Can you work these out from the model? Positions are in its coordinate system, mm. Face numbers are marked on the shaded views. A direction names the side the tool comes from. Give positions to 0.01 mm unless a question says otherwise; leave off trailing zeros. Write each loop counter-clockwise with the first axis right and the second up, starting at its lowest first coordinate (ties: lowest second). Pieces come first, ordered by that corner, then holes.
1. Suppose I cut it at A-A (x = 0.75). Please give me the cut outline in (y, z).
2. Suppose I cut it at B-B (y = 2). Please give me the cut outline in (x, z).
3. Suppose I cut it at D-D (z = -16). Please give me the cut outline in (x, y), and give its area (3 significant figures).
4. I'm going to push flat-ended pins straight in: pin 1 (5 mm diameter, centred on y = 12.5, z = -27, fed in from +X); pin 2 (1.5 mm diameter, centred on x = 1.5, z = -4, fed in from +Y). Where does each tip first touch, or does it pass through?
5. On a 3-axis mill with a long thin cutter (end or side, diameter ignored), from which of +Z, -Z, +X, -X, +Y, -Y can I reach the whole of each face in a straight line? I mean the marked faces 1 and 2. Say none if no direction works.
6. Suppose I cut it at C-C (z = -8). Please give me the cut outline in (x, y), and give its area (3 significant figures).
7. If I drill on probe 1 along Z at (x, y) = (1.25, 1.5); probe 2 along X at (y, z) = (11.75, -13), over which ranges is the centre line in solid material (lowest first)?
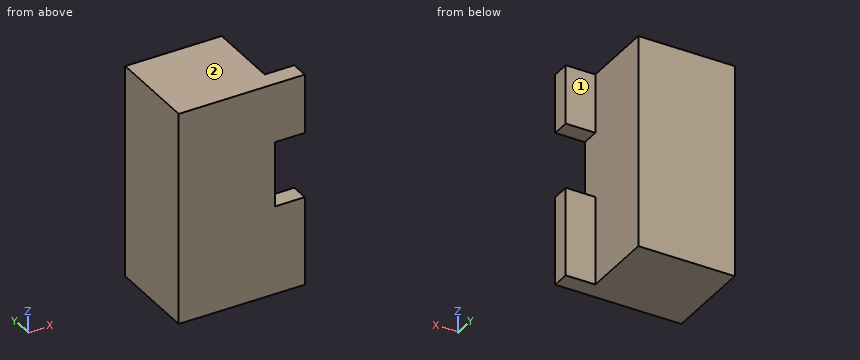
Autodesk Inventor part; units mm, degrees
ref_plane "YZ Plane" through (0, 0, 0) normal (1, 0, 0) x (0, 1, 0)
ref_plane "XZ Plane" through (0, 0, 0) normal (0, 1, 0) x (-1, 0, 0)
ref_plane "XY Plane" through (0, 0, 0) normal (0, 0, 1) x (1, 0, 0)
sketch "Sketch1" plane through (0, 0, 0) normal (0, 1, 0) x (-1, 0, 0)
  line L0 (16.3, 0) -> (0, 0)
  line L1 (0, 0) -> (0, -36)
  line L2 (0, -36) -> (16.3, -36)
  line L3 (16.3, -36) -> (16.3, 0)
  dimension "d0" = 36
  dimension "d1" = 16.3
extrude "Extrusion1" add sketch "Sketch1" along normal blind 15.3
sketch "Sketch2" plane through (0, 0, 0) normal (1, 0, 0) x (0, 0, -1)
  line L0 (0, 0) -> (0, 15.3)
  line L1 (0, 0) -> (10, 0)
  line L2 (10, 0) -> (10, 3)
  line L3 (10, 3) -> (0, 3)
  line L4 (0, 3) -> (0, 0)
  line L5 (0, 0) -> (36, 0)
  line L6 (36, 0) -> (21, 0)
  line L7 (21, 0) -> (21, 3)
  line L8 (21, 3) -> (36, 3)
  line L9 (36, 3) -> (36, 0)
  point P0 (0, 3)
  dimension "d4" = 10
  dimension "d5" = 3
  dimension "d6" = 15
extrude "Extrusion2" add sketch "Sketch2" along normal blind 5
properties part number "AC-DC transformer"
Checks:
1. outline: (0, -36) - (3, -36) - (3, -21) - (0, -21) - close; (0, -10) - (3, -10) - (3, 0) - (0, 0) - close
2. outline: (-16.3, -36) - (5, -36) - (5, -21) - (0, -21) - (0, -10) - (5, -10) - (5, 0) - (-16.3, 0) - close
3. outline: (-16.3, 0) - (0, 0) - (0, 15.3) - (-16.3, 15.3) - close
3. area: 249 mm2
4. pin 1: stops at x = 0
4. pin 2: stops at y = 3
5. face 1: +Z, -Z, +X, +Y
5. face 2: +Z, +X, -X, +Y, -Y
6. outline: (-16.3, 0) - (5, 0) - (5, 3) - (0, 3) - (0, 15.3) - (-16.3, 15.3) - close
6. area: 264 mm2
7. probe 1: z = -36 to -21, -10 to 0
7. probe 2: x = -16.3 to 0
